The listing builds one solid part. Answer for the finished solid, in the listing's coordinates (mm). A direction names the side the tool comes from. Coordinates: 2 decimals unless noted, no trailing zeros. Loops run counter-clockwise (first coordinate to the right, second up) from the corner with the lowest first, then second, coordinate; pieces in that order, holes last. Notation, with made-up numbers: M 7.5,-22 L 50.5,-22 A34 ccw 50.5,11 Z; hole C -31,52 d2. An arc over 180 degrees is marked long. Answer in a Markdown table with one row per item. Add a question column.
Autodesk Fusion 360 part; units mm, degrees
sketch "Sketch1" plane through (0, 0, 0) normal (0, 1, 0) x (1, 0, 0)
  line L0 (0, 0) -> (-88.9, 0)
  line L1 (-88.9, 0) -> (-88.9, -111.125)
  line L2 (-88.9, -111.125) -> (0, -111.125)
  line L3 (0, -111.125) -> (0, 0)
  line L4 (0, -12.7) -> (-88.9, -12.7)
  line L5 (0, -31.75) -> (-88.9, -31.75)
  line L6 (0, -88.9) -> (-88.9, -88.9)
  line L7 (0, -98.425) -> (-88.9, -98.425)
  dimension "d1" = 88.9
  dimension "d2" = 111.125
  dimension "d3" = 12.7
  dimension "d5" = 19.05
  dimension "d6" = 12.7
  dimension "d7" = 9.525
extrude "Extrude1" add sketch "Sketch1" along normal blind 25.4 contours L1 L3 L5 L6 | L1 L3 L6 L7 | L1 L2 L3 L7
extrude "Extrude2" add sketch "Sketch1" along normal blind 19.05 contours L0 L1 L3 L4 | L1 L3 L4 L5
extrude "Extrude3" cut sketch "Sketch1" along normal blind 6.35 contours L1 L3 L4 L5 | L1 L3 L6 L7
extrude "Extrude4" cut sketch "Sketch1" along normal blind 7.9375 contours L1 L3 L5 L6
fillet "Fillet1" radius 1 13 edges at (-44.45, 6.35, 98.425) (-44.45, 6.35, 88.9) (-44.45, 7.9375, 88.9) (-44.45, 7.9375, 31.75) (-44.45, 6.35, 31.75) (-44.45, 0, 12.7) (-44.45, 0, 98.425) (-44.45, 0, 0) (-44.45, 19.05, 0) (-44.45, 19.05, 31.75) (-44.45, 25.4, 31.75) (-44.45, 25.4, 111.125) (-44.45, 0, 111.125)
fillet "Fillet2" radius 1 2 faces at (0, 19.5792, 76.9393) (-88.9, 19.5792, 76.9393)
equation "d2 = 4 3/8\""
equation "d7 = 3 in / 8"
equation "d14 = 0.25 in + 1\" / 16"
(1) Each of these flat-tipped pins is pushed along its axis until it touches: pin 1 (16.5 mm diameter, centred on x = -52, z = 52, fed in from -Y); pin 2 (3.5 mm diameter, centred on x = -23.5, y = 21.5, fed in from -Z); pin 3 (8.5 mm diameter, centred on x = -24, z = 93, fed in from -Y). Where does it stop, or does it pass through?
(2) A cutting plane is placed at A-A (y = 2.5). Give the vertices of the cut face in (x, z) (3 decimals).
(3) A cutting plane is placed at C-C (y = 23). Give the vertices of the cut face in (x, z) (3 decimals), plus the area to 3 significant figures.
(4) Straight lines are drawn through the part: line 1 (Z direction, x = -26, y = 4.75) (3 decimals); line 2 (Y direction, x = -17.5, z = 47); line 3 (Y direction, x = -22.5, z = 24). For each, find the intervals that lie inside material, in ascending order.
(5) For faces 1 (the face through (-88.9, 15, 55)), 2 (the face through (-44, 22, 31.75)), 3 (the face through (-44, 4, 12.7)), determine the directions among +Z, -Z, +X, -X, +Y, -Y from which every point of the face is accessible in a straight line to the end or side of a thin tool.
(6) A cutting plane is placed at B-B (z = 64.5). Give the vertices of the cut face in (x, y).
Solved:
| question | item | result |
|---|---|---|
| 1 | pin 1 | stops at y = 7.94 |
| 1 | pin 2 | stops at z = 31.7 |
| 1 | pin 3 | stops at y = 6.35 |
| 2 | outline | M -88.9,1 A1 ccw -87.9,0 L -1,0 A1 ccw 0,1 L 0,11.7 A1 ccw -1,12.7 L -87.9,12.7 A1 ccw -88.9,11.7 Z; M -88.9,99.425 A1 ccw -87.9,98.425 L -1,98.425 A1 ccw 0,99.425 L 0,110.125 A1 ccw -1,111.125 L -87.9,111.125 A1 ccw -88.9,110.125 Z |
| 3 | outline | M -88.9,32.75 A1 ccw -87.9,31.75 L -1,31.75 A1 ccw 0,32.75 L 0,110.125 A1 ccw -1,111.125 L -87.9,111.125 A1 ccw -88.9,110.125 Z |
| 3 | area | 7,060 mm² |
| 4 | line 1 | z = 0 to 12.7, 98.425 to 111.125 |
| 4 | line 2 | y = 7.94 to 25.4 |
| 4 | line 3 | y = 6.35 to 19.05 |
| 5 | face 1 | +Z, -Z, -X, +Y, -Y |
| 5 | face 2 | -Z, +X, -X, +Y |
| 5 | face 3 | +X, -X, -Y |
| 6 | outline | M -88.9,8.94 A1 ccw -87.9,7.94 L -1,7.94 A1 ccw 0,8.94 L 0,24.4 A1 ccw -1,25.4 L -87.9,25.4 A1 ccw -88.9,24.4 Z |
